Input: part model. Units: mm. Frame: model coordinates. A direction names the side the tool comes from. Coordinates: 2 decimals unless noted, no trailing zeros. Write each loop counter-clockwise with the first axis right and the second up, starting at its lowest first coordinate (ties: lowest second). Pieces come first, ordered by that corner, then holes.
from build123d import *

# Parameters (mm, degrees)
BOSS_EXTRUDE1_DEPTH          = 1
EDGE_FLANGE1_STRIP_W         = 7
EDGE_FLANGE1_STRIP_H         = 1
EDGE_FLANGE1_STRIP_CUT_DEPTH = 36
EDGE_FLANGE1_DEPTH           = 36
SKETCH12_R                   = 1.5
CUT_EXTRUDE2_DEPTH           = 1
FILLET1_R                    = 5


# Sheet-metal steps are written as plain solids
with BuildPart() as part:
    # Sketch1 → Boss-Extrude1 (new body)
    with BuildSketch(Plane.XY):
        with BuildLine():
            Line((11.5, 10), (12.5, 10))
            ThreePointArc((12.5, 10), (12.911299923, 11.031858587), (13.919642857, 11.49784603))
            ThreePointArc((13.919642857, 11.49784603), (9.899494937, 19.899494937), (1.49784603, 23.919642857))
            ThreePointArc((1.49784603, 23.919642857), (0, 22.5), (-1.49784603, 23.919642857))
            ThreePointArc((-1.49784603, 23.919642857), (-9.899494937, 19.899494937), (-13.919642857, 11.49784603))
            ThreePointArc((-13.919642857, 11.49784603), (-12.911299923, 11.031858587), (-12.5, 10))
            Line((-12.5, 10), (-11.5, 10))
            ThreePointArc((-11.5, 10), (0, 21.5), (11.5, 10))
        make_face()
        with BuildLine():
            ThreePointArc((13.919642857, 11.49784603), (15.031858587, 11.088700077), (15.5, 10))
            Line((15.5, 10), (18, 10))
            ThreePointArc((18, 10), (0, 28), (-18, 10))
            Line((-18, 10), (-15.5, 10))
            ThreePointArc((-15.5, 10), (-15.031858587, 11.088700077), (-13.919642857, 11.49784603))
            ThreePointArc((-13.919642857, 11.49784603), (-9.899494937, 19.899494937), (-1.49784603, 23.919642857))
            ThreePointArc((-1.49784603, 23.919642857), (-0.040193003, 25.499461411), (1.5, 24))
            ThreePointArc((1.5, 24), (1.499461411, 23.959806997), (1.49784603, 23.919642857))
            ThreePointArc((1.49784603, 23.919642857), (9.899494937, 19.899494937), (13.919642857, 11.49784603))
        make_face()
        with BuildLine():
            ThreePointArc((13.919642857, 8.50215397), (12.911299923, 8.968141413), (12.5, 10))
            Line((12.5, 10), (11.5, 10))
            ThreePointArc((11.5, 10), (0, -1.5), (-11.5, 10))
            Line((-11.5, 10), (-12.5, 10))
            ThreePointArc((-12.5, 10), (-12.911299923, 8.968141413), (-13.919642857, 8.50215397))
            ThreePointArc((-13.919642857, 8.50215397), (-9.899494937, 0.100505063), (-1.49784603, -3.919642857))
            ThreePointArc((-1.49784603, -3.919642857), (0, -2.5), (1.49784603, -3.919642857))
            ThreePointArc((1.49784603, -3.919642857), (9.899494937, 0.100505063), (13.919642857, 8.50215397))
        make_face()
        with BuildLine():
            Line((18, 10), (15.5, 10))
            ThreePointArc((15.5, 10), (15.031858587, 8.911299923), (13.919642857, 8.50215397))
            ThreePointArc((13.919642857, 8.50215397), (9.899494937, 0.100505063), (1.49784603, -3.919642857))
            ThreePointArc((1.49784603, -3.919642857), (1.499461411, -3.959806997), (1.5, -4))
            ThreePointArc((1.5, -4), (-0.040193003, -5.499461411), (-1.49784603, -3.919642857))
            ThreePointArc((-1.49784603, -3.919642857), (-9.899494937, 0.100505063), (-13.919642857, 8.50215397))
            ThreePointArc((-13.919642857, 8.50215397), (-15.031858587, 8.911299923), (-15.5, 10))
            Line((-15.5, 10), (-18, 10))
            ThreePointArc((-18, 10), (0, -8), (18, 10))
        make_face()
        with BuildLine():
            Line((18, -10), (18, 10))
            ThreePointArc((18, 10), (0, -8), (-18, 10))
            Line((-18, 10), (-18, -10))
            Line((-18, -10), (18, -10))
        make_face()
    extrude(amount=BOSS_EXTRUDE1_DEPTH)

    # Edge-Flange1 strip (across the edge) → Edge-Flange1 strip cut (cut)
    with BuildSketch(Plane(origin=(18, -10, 0), x_dir=(0, 1, 0), z_dir=(-1, 0, 0))):
        with Locations((-1, -0.5)):
            Rectangle(EDGE_FLANGE1_STRIP_W, EDGE_FLANGE1_STRIP_H)
    extrude(amount=EDGE_FLANGE1_STRIP_CUT_DEPTH, mode=Mode.SUBTRACT)

    # Edge-Flange1 section (across the edge) → Edge-Flange1 (add)
    with BuildSketch(Plane(origin=(18, -10, 0), x_dir=(0, 1, 0), z_dir=(-1, 0, 0))):
        with BuildLine():
            Line((0, 1.5), (0, 69))
            Line((0, 69), (1, 69))
            Line((1, 69), (1, 1.5))
            ThreePointArc((1, 1.5), (1.439339828, 0.439339828), (2.5, 0))
            Line((2.5, 0), (2.5, -1))
            ThreePointArc((2.5, -1), (0.732233047, -0.267766953), (0, 1.5))
        make_face()
    extrude(amount=EDGE_FLANGE1_DEPTH)

    # Sketch12 → Cut-Extrude2 (cut)
    with BuildSketch(Plane(origin=(0, -9, 0), x_dir=(1, 0, 0), z_dir=(0, 1, 0))):
        with BuildLine():
            Line((-18, 69), (-18, 1.5))
            Line((-18, 1.5), (-13.335935783, 5.66873596))
            ThreePointArc((-13.335935783, 5.66873596), (-10.872003446, 9.040546507), (-10, 13.124622769))
            Line((-10, 13.124622769), (-10, 69))
            Line((-10, 69), (-18, 69))
        make_face()
        with BuildLine():
            Line((13.335935783, 5.66873596), (18, 1.5))
            Line((18, 1.5), (18, 69))
            Line((18, 69), (10, 69))
            Line((10, 69), (10, 13.124622769))
            ThreePointArc((10, 13.124622769), (10.872003446, 9.040546507), (13.335935783, 5.66873596))
        make_face()
        with Locations(Location((-6, 64, 0), (0, 0, 270))):
            Circle(SKETCH12_R)
        with Locations(Location((6, 64, 0), (0, 0, 270))):
            Circle(SKETCH12_R)
        with Locations(Location((-6, 49, 0), (0, 0, 270))):
            Circle(SKETCH12_R)
        with Locations(Location((6, 49, 0), (0, 0, 270))):
            Circle(SKETCH12_R)
        with Locations(Location((-6, 34, 0), (0, 0, 270))):
            Circle(SKETCH12_R)
        with Locations(Location((6, 34, 0), (0, 0, 270))):
            Circle(SKETCH12_R)
        with Locations(Location((-6, 9, 0), (0, 0, 270))):
            Circle(SKETCH12_R)
        with Locations(Location((6, 9, 0), (0, 0, 90))):
            Circle(SKETCH12_R)
    extrude(amount=-CUT_EXTRUDE2_DEPTH, mode=Mode.SUBTRACT)

    # Fillet1
    fillet1_edges = [part.edges().sort_by_distance(p)[0] for p in [
        (10, -9.5, -69),
        (-10, -9.5, -69),
    ]]
    fillet(fillet1_edges, radius=FILLET1_R)


solid = part.part
Item 1: Material intervals for line 1 (X direction, y = -9.7, z = -34); line 2 (Y direction, x = 3, z = -7); line 3 (Z direction, x = 5.5, y = -0.5), sorted ascending.
Item 2: Pull-direction query (Z, two-part tool) for faces 1 (the face through (0.252, -9.248, 0.287)), 2 (the face through (-5.55, -9.49, -62.57)), 3 (the face through (-10.896, -9.493, -8.987)); classes: released by +Z, released by -Z, zero draft, split by the parting line, or undercut.
Item 3: Section query C-C, the plane z = -9. Return loops of the section in (x, y), then the cut area to 3 significant figures.
Item 4: Access query for faces 4 (the face through (0, -9, -36)), 5 (the face through (0, -10, -35)). Directions: +Z, -Z, +X, -X, +Y, -Y. A direction counts if a zero-diameter tool reaches every point of the face in a straight line with its end or side. Return the directions, or none.
Item 5: Pin query (flat end, axial travel): pin 1 Ø10 at (x, y) = (-7, 14.5) entering from -Z; pin 2 Ø0.5 at (y, z) = (-9.5, -28) entering from -X; pin 3 Ø2.5 at (x, z) = (6, -64) entering from -Y; pin 4 Ø3.5 at (x, z) = (-6, -9) entering from +Y. Return the tip coordinate at first contact, or that it passes through.
Item 6: Section query B-B, the plane y = 19. Return loops of the section in (x, z), then the cut area to 3 significant figures.
Item 7: Section query D-D, the plane z = -23.5. Return loops of the section in (x, y).
Item 8: Section query A-A, the plane z = -49. Return loops of the section in (x, y), then the cut area to 3 significant figures.
The answers:
1. line 1: x = -10 to -7.5, -4.5 to 4.5, 7.5 to 10
1. line 2: y = -10 to -9
1. line 3: z = 0 to 1
2. face 1: released by +Z
2. face 2: undercut
2. face 3: released by -Z
3. outline: (-10.89, -10) - (-7.5, -10) - (-7.5, -9) - (-10.89, -9) - close; (-4.5, -10) - (4.5, -10) - (4.5, -9) - (-4.5, -9) - close; (7.5, -10) - (10.89, -10) - (10.89, -9) - (7.5, -9) - close
3. area: 15.8 mm2
4. face 4: -Z, +X, -X, +Y
4. face 5: +Z, -Z, +X, -X, -Y
5. pin 1: stops at z = 0
5. pin 2: stops at x = -10
5. pin 3: passes through
5. pin 4: stops at y = -9
6. outline: (-15.59, 0) - (-7.16, 0) - (-7.16, 1) - (-15.59, 1) - close; (7.16, 0) - (15.59, 0) - (15.59, 1) - (7.16, 1) - close
6. area: 16.9 mm2
7. outline: (-10, -10) - (10, -10) - (10, -9) - (-10, -9) - close
8. outline: (-10, -10) - (-7.5, -10) - (-7.5, -9) - (-10, -9) - close; (-4.5, -10) - (4.5, -10) - (4.5, -9) - (-4.5, -9) - close; (7.5, -10) - (10, -10) - (10, -9) - (7.5, -9) - close
8. area: 14.0 mm2
